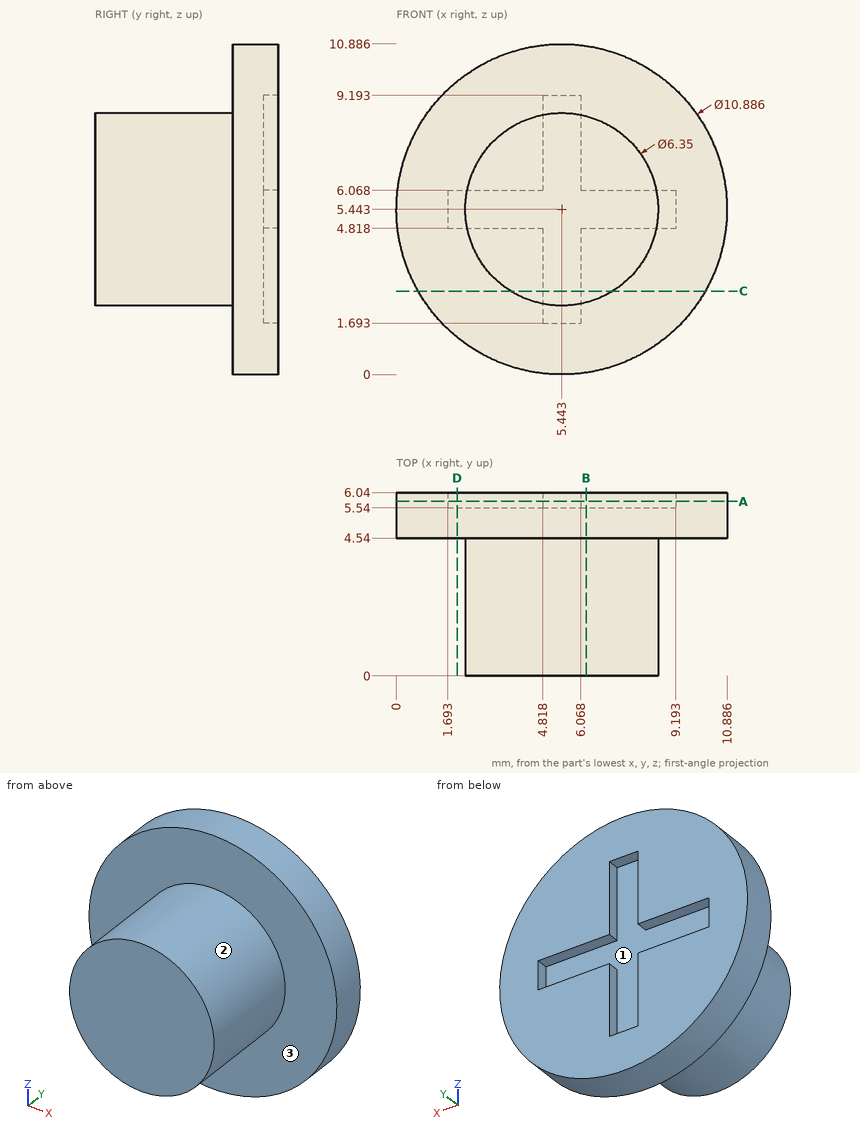
Geometry check sheet. Reference: drawing and pictorial views, mm from the part's lowest x, y, z. Coordinates: 2 decimals unless noted, no trailing zeros. Order: outer loops, then holes, each group sorted by start corner. A loop starts at its lowest first (then second) coordinate and runs counter-clockwise, first axis right, second up. Notation, with made-up numbers: (76.5, 72.25) -> (113.5, 72.25) arc R22 ccw to (113.5, 78.25) -> close; hole circle Ø7 at (17.5, 72). An arc over 180 degrees is marked (long way). Use CSV: the item, a comma, the result in double quotes. Start each with the question number.
Q1. Section check B-B, the plane x = 6.25. Record the cut outline in (y, z).
Q2. Thickness scan on line 1 along Y through (x, z) = (9, 8.75); line 2 along Y through (x, z) = (6, 8.75); line 3 along Z through (x, y) = (1.75, 5.75) (1 decimal). Record the ranges inside material, lowest first.
Q3. Section check A-A, the plane y = 5.75. Record the cut outline in (x, z).
Q4. Section check C-C, the plane z = 2.75. Record the cut outline in (x, y) (1 decimal).
Q5. Depth check by flat-ended pin: P1, Ø5.5, axis at x = 4.5, z = 6, coming from the -Y side; P2, Ø1, axis at x = 2, z = 3, coming from the -Y side; P3, Ø1.5, axis at x = 7.5, y = 4, coming from the +Z side; P4, Ø0.6, axis at y = 6, z = 7.5, coming from the +X side. Enter the tip coordinate at first touch or a pass-through.
Q6. Section check D-D, the plane x = 2. Record the cut outline in (y, z), and give its area (3 significant figures).
Q7. Draft check along X on the marked faces 1, 2 and 3. Enter one of: +X half, -X half, draft (parallel to the pull), parting line (faces both ways), or undercut.
Returned:
1,outline,"(0, 2.37) -> (4.54, 2.37) -> (4.54, 0.06) -> (6.04, 0.06) -> (6.04, 4.82) -> (5.54, 4.82) -> (5.54, 6.07) -> (6.04, 6.07) -> (6.04, 10.83) -> (4.54, 10.83) -> (4.54, 8.51) -> (0, 8.51) -> close"
2,line 1,"y = 4.54 to 6.04"
2,line 2,"y = 4.54 to 5.54"
2,line 3,"z = 1.4 to 4.8, 6.1 to 9.4"
3,outline,"circle Ø10.89 at (5.44, 5.44); hole (1.69, 4.82) -> (4.82, 4.82) -> (4.82, 1.69) -> (6.07, 1.69) -> (6.07, 4.82) -> (9.19, 4.82) -> (9.19, 6.07) -> (6.07, 6.07) -> (6.07, 9.19) -> (4.82, 9.19) -> (4.82, 6.07) -> (1.69, 6.07) -> close"
4,outline,"(0.7, 4.5) -> (3.8, 4.5) -> (3.8, 0) -> (7.1, 0) -> (7.1, 4.5) -> (10.2, 4.5) -> (10.2, 6) -> (6.1, 6) -> (6.1, 5.5) -> (4.8, 5.5) -> (4.8, 6) -> (0.7, 6) -> close"
5,P1,"stops at y = 0"
5,P2,"stops at y = 4.54"
5,P3,"stops at z = 10.66"
5,P4,"stops at x = 10.59"
6,outline,"(4.54, 1.23) -> (6.04, 1.23) -> (6.04, 4.82) -> (5.54, 4.82) -> (5.54, 6.07) -> (6.04, 6.07) -> (6.04, 9.66) -> (4.54, 9.66) -> close"
6,area,"12.0 mm^2"
7,face 1,"undercut"
7,face 2,"parting line"
7,face 3,"draft"
